Answer from the drawing. Dimensions are ordinates in mm from the lowest x, y and z of the part. Round coordinates to 2 decimals unless told otherwise and drop trailing zeros. Write each loop counter-clockwise with the first axis right and the second up, starting at its lowest first coordinate (ties: lowest second). Pieces come first, ordered by that corner, then holes. Notation, with made-up numbers: (-23, 86.25) - (30, 86.25) arc R4 cw to (30, 92.25) - close; hole circle Ø10 at (60.5, 13). An arc over 180 degrees is marked (long way). Answer in a Markdown table with one row per item.
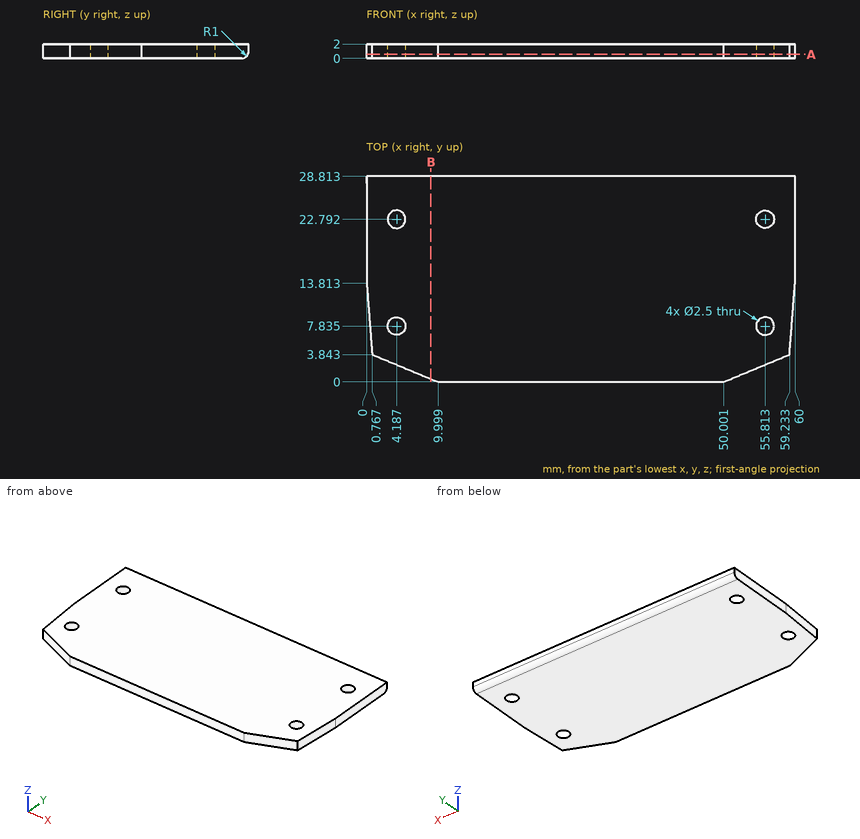
(1) Section B-B (x = 9) is taken. Give the vertices of the cut face in (y, z) (1 decimal).
Checked values:
| item | result |
|---|---|
| outline | (0.4, 0) - (27.8, 0) arc R1 ccw to (28.8, 1) - (28.8, 2) - (0.4, 2) - close |
(2) Find the intervals of material crossed by line 1 (X direction, y = 8.5, z = 1.4) (1 decimal); line 2 (X direction, y = 22.25, z = 1.1) (1 decimal); line 3 (X direction, y = 11.5, z = 0.8), in increasing order.
Checked values:
| item | result |
|---|---|
| line 1 | x = 0.4 to 3.1, 5.2 to 54.8, 56.9 to 59.6 |
| line 2 | x = 0 to 3.1, 5.3 to 54.7, 56.9 to 60 |
| line 3 | x = 0.18 to 59.82 |
(3) Section A-A (z = 0.55) is taken. State how many separate pieces and enclosed holes the cut face has, and give its area (3 significant figures).
Checked values:
| item | result |
|---|---|
| separate pieces | 1 |
| enclosed holes | 4 |
| area | 1,650 mm2 |
